Can you work these out from the drawing? Everything is in mm from the part's minimum corner. Give positions to 0.01 mm unless a question says otherwise; leave off trailing zeros. Order: outer loops, then holes, each group sorted by start corner. A loop starts at its lowest first (then second) coordinate and runs counter-clockwise, first axis right, second up. Notation, with made-up numbers: (50, -9.75) - (105, -9.75) arc R21 cw to (105, 16.25) - close; hole circle Ø3 at (37.5, 89). An arc over 180 degrees is marked (long way). Answer as a JSON object with one key per item and string values.
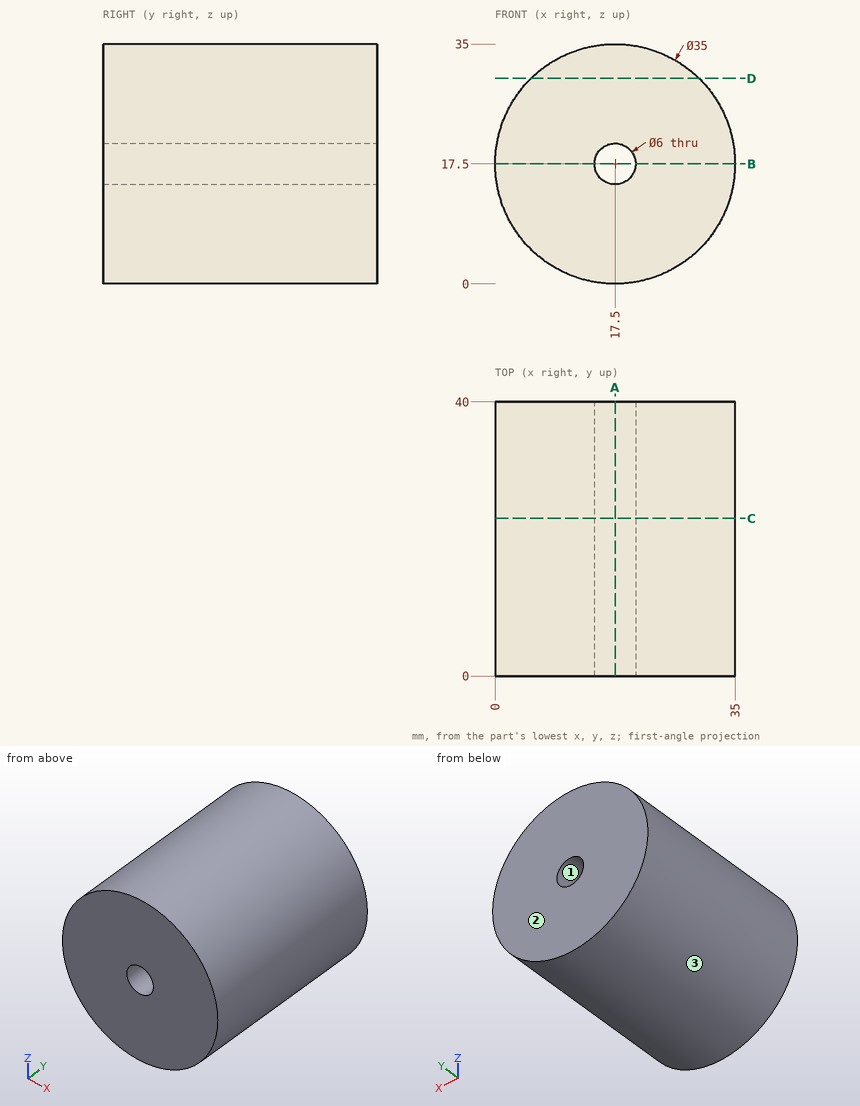
Q1. I need wall thicknesses on L1, parallel to Z at x = 17.5, y = 10.5; L2, parallel to X at y = 11, z = 15. Which ranges of each line are inside material? Lowest first, please.
Recorded:
{"L1": "z = 0 to 14.5, 20.5 to 35", "L2": "x = 0.18 to 15.84, 19.16 to 34.82"}
Q2. If we section it at A-A, the plane x = 17.5: Please give me the cut outline in (y, z).
Recorded:
{"outline": "(0, 0) - (40, 0) - (40, 14.5) - (0, 14.5) - close; (0, 20.5) - (40, 20.5) - (40, 35) - (0, 35) - close"}
Q3. I'm going to push flat-ended pins straight in: pin 1 Ø8 at (y, z) = (28.5, 7.5) entering from +X; pin 2 Ø10 at (x, y) = (24.5, 17.5) entering from -Z; pin 3 Ø4 at (y, z) = (16, 14.5) entering from -X. Where does each tip first touch, or does it pass through?
Recorded:
{"pin 1": "stops at x = 33.94", "pin 2": "stops at z = 0.11", "pin 3": "stops at x = 0.03"}
Q4. If we section it at D-D, the plane z = 30: Please give me the cut outline in (x, y), then the cut area to 3 significant figures.
Recorded:
{"outline": "(5.25, 0) - (29.75, 0) - (29.75, 40) - (5.25, 40) - close", "area": "980 mm^2"}
Q5. If we section it at B-B, the plane z = 17.5: Please give me the cut outline in (x, y).
Recorded:
{"outline": "(0, 0) - (14.5, 0) - (14.5, 40) - (0, 40) - close; (20.5, 0) - (35, 0) - (35, 40) - (20.5, 40) - close"}
Q6. If we section it at C-C, the plane y = 23: Please give me the cut outline in (x, z), then the cut area to 3 significant figures.
Recorded:
{"outline": "circle Ø35 at (17.5, 17.5); hole circle Ø6 at (17.5, 17.5)", "area": "934 mm^2"}
Q7. We'd pull the mould along X, two halves only. Please class the marked faces 1, 2 and 3: released by +X, released by -X, zero draft, split by the parting line, or undercut.
Recorded:
{"face 1": "undercut", "face 2": "zero draft", "face 3": "split by the parting line"}
